For this review, take the finished solid that the model builds, in its own axes (mm). A direction names the side the tool comes from. Round coordinates to 2 decimals unless told otherwise and drop trailing zeros. Loops run counter-clockwise (first coordinate to the right, second up) from the corner with the lowest first, then second, coordinate; pieces in that order, holes last.
1) Wall thickness on L1, parallel to Y at x = -4.5, z = 0.75; L2, parallel to Y at x = -27.5, z = 0.7; L3, parallel to X at y = 14, z = 2.45: over which ranges is each line inside the solid? List them lowest first.
2) Insertion check: pin 1 (1 mm diameter, centred on y = 25.5, z = 3.5, fed in from -X); pin 2 (2 mm diameter, centred on x = -47, z = 3.5, fed in from -Y); pin 3 (1.5 mm diameter, centred on x = -24, z = 3, fed in from -Y). Each pin has a flat end and moves straight along its axis. Give the tip position at first contact, or say it passes through.
3) Take a section at A-A (y = 53). State the section outline as (x, z) points, then the cut area to 3 significant figures.
4) Mouldability with a two-part tool opening along Y and no side actions: class faces 4 (the flat face through (-11.497, 34.339, 2.465)), 5 (the flat face through (-32.6, 44.2, 0)), 6 (the flat face through (6, 0.3, 2.5)), 7 (the flat face through (2.785, -4.425, 2.465)) as pulls with the +Y half, pulls with the -Y half, needs draft (parallel to the pull), parting line crosses it, or undercut.
5) Tool access review of faces 1 (the cylindrical face through (0.92, 0.67, 2.46)), 2 (the flat face through (0, 34, 2)), 3 (the flat face through (-64.91, 55.19, 2.46)): name each direction out of +Z, -Z, +X, -X, +Y, -Y from which nothing blocks a thin tool from reaching the whole face with its end or side.
6) Take a section at B-B (y = 15.5). State the section outline as (x, z) points, then the cut area to 3 significant figures.
7) Take a section at C-C (x = -86.5). State the section outline as (y, z) points, then the cut area to 3 significant figures.
```python
from build123d import *

# Parameters (mm, degrees)
F1_DEPTH = 5
F2_R     = 1.5
F3_R     = 2
F4_R     = 10
F5_R     = 1


with BuildPart() as f1:
    # F0 (on Top) → F1 (new body)
    with BuildSketch(Plane.XY):
        with BuildLine():
            Line((9, 0.6), (3, 0))
            ThreePointArc((3, 0), (0.897663, 0.691907), (0, 2.714963))
            Line((0, 2.714963), (0, 66.785037))
            ThreePointArc((0, 66.785037), (0.897663, 68.808093), (3, 69.5))
            Line((3, 69.5), (9, 68.9))
            Line((9, 68.9), (8.900496, 67.904963))
            Line((8.900496, 67.904963), (10.100496, 67.904963))
            Line((10.100496, 67.904963), (10.100496, 71.5))
            Line((10.100496, 71.5), (-3, 71.5))
            Line((-3, 71.5), (-110.518552, 49.457754))
            Line((-110.518552, 49.457754), (-90.286419, 49.987845))
            Line((-90.286419, 49.987845), (-36.891579, 60.934255))
            Line((-36.891579, 60.934255), (-30.92766, 34.601165))
            Line((-30.92766, 34.601165), (-20.210214, 32.223703))
            Line((-20.210214, 32.223703), (-3, 36.40078))
            Line((-3, 36.40078), (-3, 2.552214))
            Line((-3, 2.552214), (-7.496703, 0.485405))
            Line((-7.496703, 0.485405), (-4.178624, -6.733656))
            Line((-4.178624, -6.733656), (10.100496, -2))
            Line((10.100496, -2), (10.100496, 1.595037))
            Line((10.100496, 1.595037), (8.900496, 1.595037))
            Line((8.900496, 1.595037), (9, 0.6))
        make_face()
        Polygon((-28.311197, 37.116512), (-33.84681, 61.55846), (-3, 67.882326), (-3, 39.46185), (-20.135539, 35.302897), align=None, mode=Mode.SUBTRACT)
    extrude(amount=F1_DEPTH)

    # F2
    f2_edges = [f1.edges().sort_by_distance(p)[0] for p in [
        (10.100496, 71.5, 2.5),
        (10.100496, -2, 2.5),
    ]]
    fillet(f2_edges, radius=F2_R)

    # F3
    f3_edges = [f1.edges().sort_by_distance(p)[0] for p in [
        (-3, 2.552214, 2.5),
        (-3, 39.46185, 2.5),
        (-20.135539, 35.302897, 2.5),
        (-28.311197, 37.116512, 2.5),
        (-33.84681, 61.55846, 2.5),
        (-3, 67.882326, 2.5),
        (-36.891579, 60.934255, 2.5),
        (-30.92766, 34.601165, 2.5),
        (-20.210214, 32.223703, 2.5),
    ]]
    fillet(f3_edges, radius=F3_R)

    # F4
    f4_edges = [f1.edges().sort_by_distance(p)[0] for p in [
        (-3, 71.5, 2.5),
    ]]
    fillet(f4_edges, radius=F4_R)

    # F5
    f5_edges = [f1.edges().sort_by_distance(p)[0] for p in [
        (-4.178624, -6.733656, 2.5),
        (-7.496703, 0.485405, 2.5),
    ]]
    fillet(f5_edges, radius=F5_R)


solid = f1.part
```
Response:
1. L1: y = -6.02 to 1.86, 36.04 to 39.1, 67.37 to 71.19
1. L2: y = 33.84 to 36.99, 62.86 to 66.48
1. L3: x = -3 to 0
2. pin 1: stops at x = -3
2. pin 2: stops at y = 58.66
2. pin 3: stops at y = 32.9
3. outline: (-93.24, 0) - (-75.59, 0) - (-75.59, 5) - (-93.24, 5) - close; (-35.09, 0) - (-31.91, 0) - (-31.91, 5) - (-35.09, 5) - close; (-3, 0) - (0, 0) - (0, 5) - (-3, 5) - close
3. area: 119 mm2
4. face 4: undercut
4. face 5: needs draft
4. face 6: undercut
4. face 7: pulls with the -Y half
5. face 1: +Z, -Z
5. face 2: +Z, -Z, +X
5. face 3: +Z, -Z, -Y
6. outline: (-3, 0) - (0, 0) - (0, 5) - (-3, 5) - close
6. area: 15.0 mm2
7. outline: (50.76, 0) - (54.38, 0) - (54.38, 5) - (50.76, 5) - close
7. area: 18.1 mm2
